Geometry: final body of the model. Coordinates: model frame, mm. A direction names the side the tool comes from. Give positions to 0.01 mm unless a question says otherwise; leave off trailing zeros. Loops run counter-clockwise (first coordinate to the right, second up) from the corner with the lowest first, then second, coordinate; pieces in that order, holes last.
1. Section A-A, the plane y = 10.25. State how many separate pieces and enclosed holes the cut face has, then the cut area to 3 significant figures.
2. Draft query along X for faces 1 (the face through (14.97, 2.64, -48.01)), 2 (the face through (5, 10, -7)), 3 (the face through (27, 9, -50)), 4 (the face through (23, 13, -50)). Return one class per face: +X half, -X half, draft (parallel to the pull), parting line (faces both ways), or undercut.
3. Access query for faces 5 (the face through (7.1, 8.7, -10)), 6 (the face through (5, 10, -50)), 7 (the face through (23.1, 8.7, -5)), 8 (the face through (7.1, 8.7, -52.5)). Directions: +Z, -Z, +X, -X, +Y, -Y. A direction counts if a zero-diameter tool reaches every point of the face in a straight line with its end or side. Return the directions, or none.
4. Section D-D, the plane x = 15. Output: boundary loops of the cut face in (y, z), then the cut area to 3 significant figures.
5. Section C-C, the plane y = 4. Output: boundary loops of the cut face in (x, z).
6. First-contact query: P1, Ø2.5, axis at y = 9.5, z = -49, coming from the +X side; P2, Ø4, axis at x = 8.5, y = 7.5, coming from the +Z side; P3, Ø2, axis at x = 17.5, z = -27, coming from the +Y side; P4, Ø1.9, axis at x = 15, z = -49.75, coming from the +Y side. Flat tips, straight axial feed; report the tip coordinate or a pass-through.
7. Material intervals for line 1 along Z through (x, y) = (15, 1.9); line 2 along X through (y, z) = (1.85, -49.75); line 3 along Z through (x, y) = (3.75, 11.5), sorted ascending.
8. Section B-B, the plane x = 7. Output: boundary loops of the cut face in (y, z).
Autodesk Inventor part; units mm, degrees
ref_plane "YZ Plane" through (0, 0, 0) normal (1, 0, 0) x (0, 1, 0)
ref_plane "XZ Plane" through (0, 0, 0) normal (0, 1, 0) x (-1, 0, 0)
ref_plane "XY Plane" through (0, 0, 0) normal (0, 0, 1) x (1, 0, 0)
sketch "Náčrt1" plane through (0, 0, 0) normal (0, 1, 0) x (-1, 0, 0)
  line L0 (0, 0) -> (-30, 0)
  line L1 (-30, 0) -> (-30, -55)
  line L2 (-30, -55) -> (0, -55)
  line L3 (0, -55) -> (0, 0)
  circle A0 centre (-15, -7.45) radius 1.6
  circle A1 centre (-15, -49.75) radius 1.6
  dimension "d1" = 3.2
  dimension "d2" = 3.2
  dimension "d3" = 55
  dimension "d4" = 30
  dimension "d5" = 15
  dimension "d6" = 15
  dimension "d11" = 5.25
  dimension "d12" = 7.45
extrude "Vysunutí1" add sketch "Náčrt1" along normal blind 3
sketch "Náčrt2" plane through (0, 3, 0) normal (0, 1, 0) x (1, 0, 0)
  line L0 (3, 5) -> (11, 5)
  line L1 (11, 5) -> (11, 10)
  line L2 (11, 10) -> (3, 10)
  line L3 (3, 10) -> (3, 5)
  line L4 (27, 5) -> (19, 5)
  line L5 (19, 5) -> (19, 10)
  line L6 (19, 10) -> (27, 10)
  line L7 (27, 10) -> (27, 5)
  line L8 (0, 55) -> (0, 0)
  line L9 (0, 0) -> (30, 0)
  line L10 (30, 0) -> (30, 55)
  line L11 (-2.5391, 27.5) -> (32.8549, 27.5) construction
  line L12 (3, 47.5) -> (11, 47.5)
  line L13 (11, 47.5) -> (11, 52.5)
  line L14 (11, 52.5) -> (3, 52.5)
  line L15 (3, 52.5) -> (3, 47.5)
  line L16 (19, 47.5) -> (27, 47.5)
  line L17 (27, 47.5) -> (27, 52.5)
  line L18 (27, 52.5) -> (19, 52.5)
  line L19 (19, 52.5) -> (19, 47.5)
  line L20 (30, 55) -> (0, 55)
  dimension "d15" = 3
  dimension "d16" = 8
  dimension "d17" = 5
  dimension "d18" = 5
  dimension "d19" = 5
  dimension "d20" = 3
  dimension "d21" = 8
  dimension "d22" = 5
  dimension "d23" = 5
  dimension "d24" = 8
  dimension "d25" = 2.5
  dimension "d26" = 2.5
  dimension "d27" = 8
  dimension "d28" = 5
  dimension "d29" = 3
  dimension "d30" = 3
extrude "Vysunutí2" add sketch "Náčrt2" along normal blind 10 contours L3 L2 L1 L0 | L4 L5 L6 L7 | L15 L14 L13 L12 | L19 L18 L17 L16
fillet "Zaoblení1" radius 2 20 edges at (7, 3, -10) (23, 3, -10) (7, 3, -47.5) (23, 3, -47.5) (27, 3, -50) (23, 3, -52.5) (19, 3, -50) (11, 3, -50) (7, 3, -52.5) (3, 3, -50) (3, 3, -7.5) (7, 3, -5) (19, 3, -7.5) (23, 3, -5) (11, 3, -7.5) (27, 3, -7.5) (30, 1.5, 0) (0, 1.5, 0) (30, 1.5, -55) (0, 1.5, -55)
sketch "Náčrt3" plane through (3, 13, -5) normal (0, 0, 1) x (1, 0, 0)
  line L0 (2, -2) -> (6, -2)
  line L1 (6, -2) -> (6, -4)
  line L2 (6, -4) -> (2, -4)
  line L3 (2, -4) -> (2, -2)
  line L4 (18, -2) -> (22, -2)
  line L5 (22, -2) -> (22, -4)
  line L6 (22, -4) -> (18, -4)
  line L7 (18, -4) -> (18, -2)
  line L8 (0, -8) -> (0, 0)
  line L9 (0, 0) -> (8, 0)
  line L10 (24, -8) -> (24, 0)
  point P0 (-3, -13)
  dimension "d34" = 4
  dimension "d35" = 2
  dimension "d36" = 2
  dimension "d37" = 2
  dimension "d38" = 4
  dimension "d39" = 2
  dimension "d40" = 2
extrude "Vysunutí3" cut sketch "Náčrt3" against normal blind 50
fillet "Zaoblení2" radius 0.5 16 edges at (3, 13, -7.5) (7, 13, -5) (11, 13, -7.5) (7, 13, -10) (23, 13, -5) (19, 13, -7.5) (23, 13, -10) (27, 13, -7.5) (3, 13, -50) (7, 13, -52.5) (7, 13, -47.5) (11, 13, -50) (19, 13, -50) (23, 13, -52.5) (23, 13, -47.5) (27, 13, -50)
chamfer "Zkosení1" distance 0.5 angle 45 2 edges at (16.6, 3, -7.45) (16.6, 3, -49.75)
properties part number "CableHolderMain"
Answers below:
1. separate pieces: 8
1. enclosed holes: 0
1. area: 80.0 mm2
2. face 1: undercut
2. face 2: undercut
2. face 3: +X half
2. face 4: draft
3. face 5: +X, -X, +Y
3. face 6: +Z, -Z
3. face 7: +Z, +X, -X, +Y
3. face 8: -Z, +X, -X, +Y
4. outline: (0, -55) - (3, -55) - (3, -51.85) - (2.5, -51.35) - (0, -51.35) - close; (0, -48.15) - (2.5, -48.15) - (3, -47.65) - (3, -9.55) - (2.5, -9.05) - (0, -9.05) - close; (0, -5.85) - (2.5, -5.85) - (3, -5.35) - (3, 0) - (0, 0) - close
4. area: 145 mm2
5. outline: (2.73, -52.77) - (11.27, -52.77) - (11.27, -47.23) - (2.73, -47.23) - close; (2.73, -10.27) - (11.27, -10.27) - (11.27, -4.73) - (2.73, -4.73) - close; (18.73, -52.77) - (27.27, -52.77) - (27.27, -47.23) - (18.73, -47.23) - close; (18.73, -10.27) - (27.27, -10.27) - (27.27, -4.73) - (18.73, -4.73) - close
6. P1: stops at x = 27
6. P2: stops at z = -5
6. P3: stops at y = 3
6. P4: passes through
7. line 1: z = -55 to -51.35, -48.15 to -9.05, -5.85 to 0
7. line 2: x = 0 to 13.4, 16.6 to 30
7. line 3: z = -52.5 to -47.5, -10 to -5
8. outline: (0, -55) - (3, -55) - (3, -54.5) arc R2 cw to (5, -52.5) - (9, -52.5) - (9, -47.5) - (5, -47.5) arc R2 cw to (3, -45.5) - (3, -12) arc R2 cw to (5, -10) - (9, -10) - (9, -5) - (5, -5) arc R2 cw to (3, -3) - (3, 0) - (0, 0) - close; (11, -52.5) - (12.5, -52.5) arc R0.5 ccw to (13, -52) - (13, -48) arc R0.5 ccw to (12.5, -47.5) - (11, -47.5) - close; (11, -10) - (12.5, -10) arc R0.5 ccw to (13, -9.5) - (13, -5.5) arc R0.5 ccw to (12.5, -5) - (11, -5) - close
